Check sheet for the modelled part. Datum: model origin and axes. Units: mm. Round coordinates to 2 decimals unless told otherwise and drop trailing zeros. Write each loop counter-clockwise with the first axis right and the second up, starting at its lowest first coordinate (ties: lowest second). Pieces come first, ordered by that corner, then holes. Notation, with made-up numbers: (61.25, 71) -> (116.25, 71) arc R6 cw to (116.25, 81) -> close; hole circle Ø10 at (50, 39.5). An arc over 180 degrees is marked (long way). Write item = value, one per line.
from build123d import *

# Parameters (mm, degrees)
F1_DEPTH = 6.35


# Not quite as in the source:
# - a feature names something its author has since deleted; it is built from what else it names


with BuildPart() as f1:
    # F0 (on Front) → F1 (new body)
    with BuildSketch(Plane.XZ):
        with BuildLine():
            Line((-82.3832392616, 36.3007842489), (-88.5181630436, 36.3007842489))
            ThreePointArc((-88.5181630436, 36.3007842489), (-87.6661618487, 33.1818070528), (-85.3468053884, 30.9291396569))
            ThreePointArc((-85.3468053884, 30.9291396569), (-83.1732772521, 33.2333223579), (-82.3832392616, 36.3007842489))
        make_face()
        with BuildLine():
            Line((-69.6832392616, 36.3007842489), (-75.8181630436, 36.3007842489))
            ThreePointArc((-75.8181630436, 36.3007842489), (-74.9661618487, 33.1818070528), (-72.6468053884, 30.9291396569))
            ThreePointArc((-72.6468053884, 30.9291396569), (-70.4732772521, 33.2333223579), (-69.6832392616, 36.3007842489))
        make_face()
        with BuildLine():
            Line((-56.9832392616, 36.3007842489), (-63.1181630436, 36.3007842489))
            ThreePointArc((-63.1181630436, 36.3007842489), (-62.2661618487, 33.1818070528), (-59.9468053884, 30.9291396569))
            ThreePointArc((-59.9468053884, 30.9291396569), (-57.7732772521, 33.2333223579), (-56.9832392616, 36.3007842489))
        make_face()
        with BuildLine():
            Line((-44.2832392616, 36.3007842489), (-50.4181630436, 36.3007842489))
            ThreePointArc((-50.4181630436, 36.3007842489), (-49.5661618487, 33.1818070528), (-47.2468053884, 30.9291396569))
            ThreePointArc((-47.2468053884, 30.9291396569), (-45.0732772521, 33.2333223579), (-44.2832392616, 36.3007842489))
        make_face()
        with BuildLine():
            Line((-31.5832392616, 36.3007842489), (-37.7181630436, 36.3007842489))
            ThreePointArc((-37.7181630436, 36.3007842489), (-36.8661618487, 33.1818070528), (-34.5468053884, 30.9291396569))
            ThreePointArc((-34.5468053884, 30.9291396569), (-32.3732772521, 33.2333223579), (-31.5832392616, 36.3007842489))
        make_face()
        with BuildLine():
            Line((-18.8832392616, 36.3007842489), (-25.0181630436, 36.3007842489))
            ThreePointArc((-25.0181630436, 36.3007842489), (-24.1661618487, 33.1818070528), (-21.8468053884, 30.9291396569))
            ThreePointArc((-21.8468053884, 30.9291396569), (-19.6732772521, 33.2333223579), (-18.8832392616, 36.3007842489))
        make_face()
        Polygon((-117.1290501952, 36.3007842489), (-100.1673217514, 36.3007842489), (-88.5181630436, 36.3007842489), (-82.3832392616, 36.3007842489), (-75.8181630436, 36.3007842489), (-69.6832392616, 36.3007842489), (-63.1181630436, 36.3007842489), (-56.9832392616, 36.3007842489), (-50.4181630436, 36.3007842489), (-44.2832392616, 36.3007842489), (-37.7181630436, 36.3007842489), (-31.5832392616, 36.3007842489), (-25.0181630436, 36.3007842489), (-18.8832392616, 36.3007842489), (1.4326782486, 36.3007842489), (15.6819988042, 36.3007842489), (19.9843030423, 36.3007842489), (19.9843030423, 39.4588721526), (6.4166695811, 39.4588721526), (1.4326782486, 39.4588721526), (-106.9938540459, 39.4588721526), (-120.9527105093, 39.4588721526), (-133.2595199347, 39.4588721526), (-133.2595199347, 36.3007842489), (-127.7280002832, 36.3007842489), align=None)
    extrude(amount=F1_DEPTH)


solid = f1.part
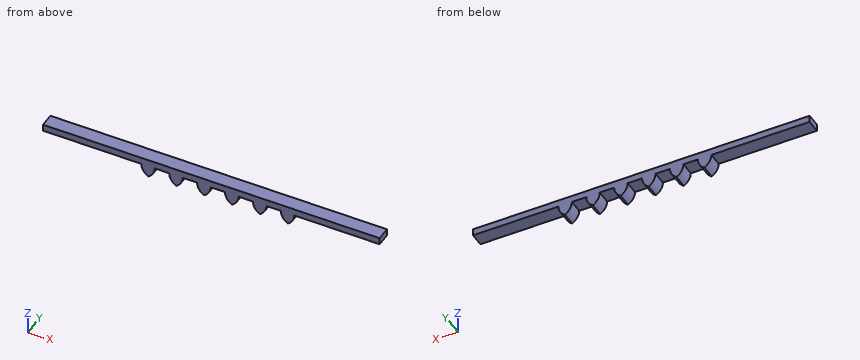
(1) Sectioned sample at A-A on y = -1. Enter the section's corners in (x, z), then the cut area to 3 significant figures.
Worked answers:
outline = (-133.26, 36.3) -> (-88.52, 36.3) arc R6.13 ccw to (-85.35, 30.93) arc R6.35 ccw to (-82.38, 36.3) -> (-75.82, 36.3) arc R6.13 ccw to (-72.65, 30.93) arc R6.35 ccw to (-69.68, 36.3) -> (-63.12, 36.3) arc R6.13 ccw to (-59.95, 30.93) arc R6.35 ccw to (-56.98, 36.3) -> (-50.42, 36.3) arc R6.13 ccw to (-47.25, 30.93) arc R6.35 ccw to (-44.28, 36.3) -> (-37.72, 36.3) arc R6.13 ccw to (-34.55, 30.93) arc R6.35 ccw to (-31.58, 36.3) -> (-25.02, 36.3) arc R6.13 ccw to (-21.85, 30.93) arc R6.35 ccw to (-18.88, 36.3) -> (19.98, 36.3) -> (19.98, 39.46) -> (-133.26, 39.46) -> close
area = 624 mm²
(2) Sectioned sample at B-B on z = 33. Enter the section's corners in (x, y).
Worked answers:
outline = (-87.55, -6.35) -> (-83.31, -6.35) -> (-83.31, 0) -> (-87.55, 0) -> close; (-74.85, -6.35) -> (-70.61, -6.35) -> (-70.61, 0) -> (-74.85, 0) -> close; (-62.15, -6.35) -> (-57.91, -6.35) -> (-57.91, 0) -> (-62.15, 0) -> close; (-49.45, -6.35) -> (-45.21, -6.35) -> (-45.21, 0) -> (-49.45, 0) -> close; (-36.75, -6.35) -> (-32.51, -6.35) -> (-32.51, 0) -> (-36.75, 0) -> close; (-24.05, -6.35) -> (-19.81, -6.35) -> (-19.81, 0) -> (-24.05, 0) -> close
(3) Sectioned sample at C-C on x = -28. Enter the section's corners in (y, z), then the cut area to 3 significant figures.
Worked answers:
outline = (-6.35, 36.3) -> (0, 36.3) -> (0, 39.46) -> (-6.35, 39.46) -> close
area = 20.1 mm²
(4) Material ranges on L1, parallel to X at y = -3.5, z = 35.25; L2, parallel to X at y = -2, z = 35.5; L3, parallel to Z at x = -105, y = -2, recorded low to high. Write a range as [from, to].
Worked answers:
L1 = [-88.43, -82.47], [-75.73, -69.77], [-63.03, -57.07], [-50.33, -44.37], [-37.63, -31.67], [-24.93, -18.97]
L2 = [-88.47, -82.43], [-75.77, -69.73], [-63.07, -57.03], [-50.37, -44.33], [-37.67, -31.63], [-24.97, -18.93]
L3 = [36.3, 39.46]
(5) Go/stop test with flat-tipped pins: P1, Ø3, axis at x = -65, y = -4.5, coming from the -Z side; P2, Ø3, axis at y = -1.5, z = 32.5, coming from the -X side; P3, Ø2, axis at x = -17.5, z = 35, coming from the +Y side. Record where each tip stops, or that it passes through.
Worked answers:
P1 = 36.3
P2 = -88.07
P3 = through
